```python
from build123d import *

# Parameters (mm, degrees)
BOSS_EXTRUDE1_DEPTH  = 2
SKETCH2_W            = 33.02
SKETCH2_H            = 22.86
BOSS_EXTRUDE2_DEPTH  = 10
M3_CLEARANCE_HOLE1_D = 3.4


with BuildPart() as part:
    # Sketch1 → Boss-Extrude1 (new body)
    with BuildSketch(Plane(origin=(0, 0, 0), x_dir=(1, 0, 0), z_dir=(0, 1, 0))):
        with BuildLine():
            Line((24.5, 46), (-24.5, 46))
            ThreePointArc((-24.5, 46), (-26.974873734, 44.974873734), (-28, 42.5))
            Line((-28, 42.5), (-28, -42.5))
            ThreePointArc((-28, -42.5), (-26.974873734, -44.974873734), (-24.5, -46))
            Line((-24.5, -46), (24.5, -46))
            ThreePointArc((24.5, -46), (26.974873734, -44.974873734), (28, -42.5))
            Line((28, -42.5), (28, 42.5))
            ThreePointArc((28, 42.5), (26.974873734, 44.974873734), (24.5, 46))
        make_face()
    extrude(amount=BOSS_EXTRUDE1_DEPTH)

    # Sketch2 → Boss-Extrude2 (add)
    with BuildSketch(Plane.XZ):
        with Locations((3.87, 26.95)):
            Rectangle(SKETCH2_W, SKETCH2_H)
    extrude(amount=-BOSS_EXTRUDE2_DEPTH)

    # M3 Clearance Hole1 (through all)
    with Locations(Plane(origin=(0, 0, 0), x_dir=(-1, 0, 0), z_dir=(0, -1, 0))):
        with Locations((-24.5, -42.5), (24.5, -42.5), (24.5, -16.5), (-24.5, -16.5), (-24.5, 42.5), (24.5, 42.5)):
            Hole(M3_CLEARANCE_HOLE1_D / 2)


solid = part.part
```
CAD build for the part. Positions are in the model's coordinates, mm. A direction names the side the tool comes from. Give positions to 0.01 mm unless a question says otherwise; leave off trailing zeros. Loops run counter-clockwise (first coordinate to the right, second up) from the corner with the lowest first, then second, coordinate; pieces in that order, holes last. Notation, with made-up numbers: M -14.75,-38 L 10.25,-38 A33 cw 10.25,0 Z; hole C 67,69 d5. An arc over 180 degrees is marked long. Use one line per item in the form item = value.
Item 1: Flat gauge pins, fed straight in: pin 1 (2.5 mm diameter, centred on x = -24.5, z = 42.5, fed in from -Y); pin 2 (17 mm diameter, centred on x = -7.5, z = 3, fed in from +Y); pin 3 (2.5 mm diameter, centred on y = 4.5, z = 29, fed in from -X); pin 4 (4 mm diameter, centred on x = 7, y = 4.5, fed in from +Z). Where does each tip first touch, or does it go through?
Determined:
pin_1 = through
pin_2 = 2
pin_3 = -12.64
pin_4 = 38.38
Item 2: Two-plate mould, pull along X, no slides. Class faces 4 (the face through (-23.7, 1, 44)), 5 (the face through (0, 1, -46)), 6 (the face through (-22.93, 1.01, 17.15)), 7 (the face through (26.95, 0.99, 45)): pulls with the +X half, pulls with the -X half, needs draft (parallel to the pull), parting line crosses it, or undercut.
Determined:
face_4 = undercut
face_5 = needs draft
face_6 = undercut
face_7 = pulls with the +X half
Item 3: Which spindle directions (+Z, -Z, +X, -X, +Y, -Y) get a long thin tool onto all of the face, cutting with end or side? Do faces 1 (the face through (4, 6, 38.38)), 2 (the face through (-12.64, 6, 27)), 3 (the face through (4, 6, 15.52)). Say none if no direction does.
Determined:
face_1 = +Z, +X, -X, +Y
face_2 = +Z, -Z, -X, +Y
face_3 = -Z, +X, -X, +Y
Item 4: Slice it at A-A (x = 4). List the corners of the cut face in (y, z), plus the area to 3 significant figures.
Determined:
outline = M 0,-46 L 2,-46 L 2,15.52 L 10,15.52 L 10,38.38 L 2,38.38 L 2,46 L 0,46 Z
area = 367 mm2
Item 5: Slice it at C-C (y = 9). List the corners of the cut face in (x, z), plus the area to 3 significant figures.
Determined:
outline = M -12.64,15.52 L 20.38,15.52 L 20.38,38.38 L -12.64,38.38 Z
area = 755 mm2
Item 6: Slice it at B-B (z = -13). List the corners of the cut face in (x, y).
Determined:
outline = M -28,0 L 28,0 L 28,2 L -28,2 Z
Item 7: Drill centre lines: probe 1 along X at (y, z) = (0.9, -42.5); probe 2 along Z at (x, y) = (-24.5, 0.5); probe 3 along Y at (x, z) = (0, -34). Where is each one in solid material? Low to high. Write a range as from..to.
Determined:
probe_1 = -28..-26.2, -22.8..22.8, 26.2..28
probe_2 = -46..-44.2, -40.8..14.8, 18.2..40.8, 44.2..46
probe_3 = 0..2
